Can you work these out from the model? Positions are in its coordinate system, mm. Round coordinates to 2 decimals unless told otherwise and drop trailing zeros. Order: outer loops, then holes, each group sorted by start corner. A loop starts at its lowest first (then second) coordinate and runs counter-clockwise, first axis right, second up. Notation, with made-up numbers: (31, 21) -> (80, 21) arc R21 ccw to (80, 29) -> close; hole circle Ø2 at (14, 33.25). An arc over 180 degrees is marked (long way). One line per item, written item: value.
```python
from build123d import *

# Parameters (mm, degrees)
F0_R     = 2.38125
F1_DEPTH = 4.699
F3_R     = 1.0922
F4_DEPTH = 7.62
F6_R     = 1.0922
F7_DEPTH = 7.62


with BuildPart() as f1:
    # F0 (on Right) → F1 (new body)
    with BuildSketch(Plane.YZ):
        with BuildLine():
            ThreePointArc((-3.753217, -9.601424), (-3.013341, -10.433085), (-1.988901, -10.868518))
            ThreePointArc((-1.988901, -10.868518), (0, -11.049), (1.988901, -10.868518))
            ThreePointArc((1.988901, -10.868518), (3.013341, -10.433085), (3.753217, -9.601424))
            Line((3.753217, -9.601424), (6.942294, -3.848176))
            ThreePointArc((6.942294, -3.848176), (6.839181, 4.028586), (0, 7.9375))
            ThreePointArc((0, 7.9375), (-6.839181, 4.028586), (-6.942294, -3.848176))
            Line((-6.942294, -3.848176), (-3.753217, -9.601424))
        make_face()
        Circle(F0_R, mode=Mode.SUBTRACT)
    extrude(amount=-F1_DEPTH)

    # F3 (on face) → F4 (cut)
    with BuildSketch(Plane(origin=(0, -5.61266, 5.61266), x_dir=(1, 0, 0), z_dir=(0, -0.707107, 0.707107))):
        with Locations((-2.286, 0)):
            Circle(F3_R)
    extrude(amount=-F4_DEPTH, mode=Mode.SUBTRACT)

    # F6 (on face) → F7 (cut)
    with BuildSketch(Plane(origin=(0, 5.61266, 5.61266), x_dir=(1, 0, 0), z_dir=(0, 0.707107, 0.707107))):
        with Locations((-2.286, 0)):
            Circle(F6_R)
    extrude(amount=-F7_DEPTH, mode=Mode.SUBTRACT)


solid = f1.part
```
Q1. Will these pins go through, and if not, where does the flat tip stop? pin 1 Ø1.5 at (x, y) = (-1.5, 6) entering from +Z; pin 2 Ø7.5 at (y, z) = (0, 0) entering from +X; pin 3 Ø2 at (x, z) = (-1, 4) entering from +Y.
Answers below:
pin 1: z = 5.93
pin 2: x = 0
pin 3: y = 7.35
Q2. Please list where these lines run through material, in increasing order: line 1 along Z through (x, y) = (-3.5, 0); line 2 along Z through (x, y) = (-2.4, 2); line 3 along Y through (x, z) = (-0.9, 1.5).
Answers below:
line 1: -11.05 to -2.38, 2.38 to 7.94
line 2: -10.87 to -1.29, 3.54 to 7.68
line 3: -7.79 to -1.85, 1.85 to 7.79
Q3. We'd pull the mould along Y, two halves only. Please class faces 1 (the face through (-2.317, -5.37, -6.685)), 2 (the face through (-2.32, 1.1, -2.11)), 3 (the face through (-4.699, 0, -4)): released by +Y, released by -Y, zero draft, split by the parting line, or undercut.
Answers below:
face 1: released by -Y
face 2: undercut
face 3: zero draft
Q4. I want a section at A-A on z = 0. List the corners of the cut face in (x, y) for me.
Answers below:
outline: (-4.7, -7.94) -> (0, -7.94) -> (0, -2.38) -> (-4.7, -2.38) -> close; (-4.7, 2.38) -> (0, 2.38) -> (0, 7.94) -> (-4.7, 7.94) -> close
Q5. I want a section at D-D on z = 4.5. Give the number of separate pieces and of enclosed holes in the cut face, plus the area to 3 significant figures.
Answers below:
separate pieces: 1
enclosed holes: 2
area: 50.9 mm^2
Q6. I want a section at C-C on x = -2.3. List the corners of the cut face in (y, z) for me (1 decimal).
Answers below:
outline: (-6.9, -3.8) -> (-3.8, -9.6) arc R2.5 ccw to (-2, -10.9) arc R11 ccw to (2, -10.9) arc R2.5 ccw to (3.8, -9.6) -> (6.9, -3.8) arc R7.9 ccw to (6.3, 4.8) -> (2.3, 0.7) arc R2.4 cw (long way) to (-2.3, 0.7) -> (-6.3, 4.8) arc R7.9 ccw to start; (-4.8, 6.3) -> (-0.7, 2.3) arc R2.4 cw to (0.7, 2.3) -> (4.8, 6.3) arc R7.9 ccw to start
Q7. I want a section at B-B on x = -3.6. List the corners of the cut face in (y, z) for me (1 decimal).
Answers below:
outline: (-6.9, -3.8) -> (-3.8, -9.6) arc R2.5 ccw to (-2, -10.9) arc R11 ccw to (2, -10.9) arc R2.5 ccw to (3.8, -9.6) -> (6.9, -3.8) arc R7.9 ccw (long way) to start; hole circle Ø4.8 at (0, 0)
